The listing builds one solid part. Answer for the finished solid, in the listing's coordinates (mm). A direction names the side the tool comes from. Give positions to 0.01 mm unless a question says otherwise; leave off trailing zeros. Loops run counter-clockwise (first coordinate to the right, second up) from the corner with the lowest first, then second, coordinate; pieces in that order, holes last. Notation, with made-up numbers: M 64,0.25 L 110,0.25 A19 cw 110,18.25 Z; hole C 88,28 d10. An arc over 180 degrees is marked long. One line per item, written item: value. Start each with the question number.
Q1. Flat-ended cylindrical pins translate along their axes: pin 1 (0.5 mm diameter, centred on x = -13, y = 32, fed in from +Z); pin 2 (0.8 mm diameter, centred on x = 112.5, y = 6.5, fed in from -Z). Find the tip coordinate at first contact, or state that the pin passes through.
Q2. For faces 4 (the flat face through (42, 31.143, 4)), 5 (the flat face through (41, 32.768, 0)), determine the directions among +Z, -Z, +X, -X, +Y, -Y from which every point of the face is accessible in a straight line to the end or side of a thin tool.
Q3. The mould has two halves that part along X. Classify faces 1 (the flat face through (117.416, 6, 0)), 2 (the flat face through (41, 7, -25)), 3 (the flat face through (42, -18.794, 4)): +X half, -X half, draft (parallel to the pull), parting line (faces both ways), or undercut.
Q4. A cutting plane is placed at C-C, the plane y = 24. Determine the outline of the cut face in (x, z), and give its area (3 significant figures).
Q5. Consider L1, parallel to Y at x = 104.5, z = 12; L2, parallel to Z at x = 64.5, y = 27.5; L3, parallel to X at y = -1.5, z = 22.5. Determine where each line is inside the solid, lowest interval first.
Q6. A cutting plane is placed at D-D, the plane x = -11.5. Determine the outline of the cut face in (y, z).
Q7. A cutting plane is placed at B-B, the plane z = 17. State how many separate pieces and enclosed holes the cut face has, and give its area (3 significant figures).
Q8. A cutting plane is placed at A-A, the plane x = 88. Determine the outline of the cut face in (y, z), and give its area (3 significant figures).
from build123d import *

# Parameters (mm, degrees)
SKETCH_1_W                = 150
SKETCH_1_H                = 53.201915286
EXTRUDE_1_DEPTH           = 25
CUT_EXTRUDE_4_DEPTH       = 132.308761728
CUT_EXTRUDE_4_DEPTH_BACK  = 132.308761728
SKETCH_2_W                = 13.960564471
SKETCH_2_H                = 10.187423892
SKETCH_2_W_2              = 14
SKETCH_2_W_3              = 12
SKETCH_2_H_2              = 5
SKETCH_4_W                = 147.277496434
SKETCH_4_H                = 49.937069792
CUT_EXTRUDE_9_DEPTH       = 40
EXTRUDE_2_DEPTH           = 0.1
EXTRUDE_2_DEPTH_BACK      = 2
SKETCH_6_W                = 147.277496434
SKETCH_6_H                = 49.937069792
CUT_EXTRUDE_11_DEPTH      = 132.012543018
CUT_EXTRUDE_11_DEPTH_BACK = 0.1
SKETCH_7_R                = 0.5


with BuildPart() as part:
    # 草图1 → 凸台-拉伸1 (new, symmetric)
    with BuildSketch(Plane.XY):
        with Locations((42.416128008, 6.167004021)):
            Rectangle(SKETCH_1_W, SKETCH_1_H)
    extrude(amount=EXTRUDE_1_DEPTH, both=True)

    # 草图2 → 切除-拉伸4 (cut, two sides: drawn at the far end of the back side and taken through both)
    with BuildSketch(Plane(origin=(0, 32.767961664, 0), x_dir=(1, 0, 0), z_dir=(0, 1, 0)).offset(-CUT_EXTRUDE_4_DEPTH_BACK)):
        with Locations((-15.114618297, -19.093711946)):
            Rectangle(SKETCH_2_W, SKETCH_2_H)
        with Locations((5.995879761, -19.093711946)):
            Rectangle(SKETCH_2_W_2, SKETCH_2_H)
        with Locations((99.312670009, -16.792388629)):
            Rectangle(SKETCH_2_W_3, SKETCH_2_H_2)
    extrude(amount=CUT_EXTRUDE_4_DEPTH + CUT_EXTRUDE_4_DEPTH_BACK, mode=Mode.SUBTRACT)

    # 草图4 → 切除-拉伸9 (cut)
    with BuildSketch(Plane.XY.offset(25)):
        with Locations((42.684765752, 6.174377474)):
            Rectangle(SKETCH_4_W, SKETCH_4_H)
    extrude(amount=-CUT_EXTRUDE_9_DEPTH, mode=Mode.SUBTRACT)

    # 草图6 → 凸台-拉伸2 (add, two sides: drawn at the far end of the back side and taken through both)
    with BuildSketch(Plane.XY.offset(25).offset(-EXTRUDE_2_DEPTH_BACK)):
        with Locations((42.684765752, 6.174377474)):
            Rectangle(SKETCH_6_W, SKETCH_6_H)
    extrude(amount=EXTRUDE_2_DEPTH + EXTRUDE_2_DEPTH_BACK)

    # 草图7 → 切除-拉伸11 (cut, two sides: drawn at the far end of the back side and taken through both)
    with BuildSketch(Plane(origin=(0, 0, 23), x_dir=(-1, 0, 0), z_dir=(0, 0, -1)).offset(-CUT_EXTRUDE_11_DEPTH_BACK)):
        with Locations((-112.698705999, 6.167004021)):
            Circle(SKETCH_7_R)
        with Locations((27.866449983, 6.174377474)):
            Circle(SKETCH_7_R)
    extrude(amount=CUT_EXTRUDE_11_DEPTH + CUT_EXTRUDE_11_DEPTH_BACK, mode=Mode.SUBTRACT)


solid = part.part
Answer block:
1. pin 1: z = 25
1. pin 2: z = -25
2. face 4: none
2. face 5: +Z, -Z, +X, -X, +Y
3. face 1: +X half
3. face 2: draft
3. face 3: undercut
4. outline: M -32.58,-25 L 117.42,-25 L 117.42,25 L 116.32,25 L 116.32,25.1 L -30.95,25.1 L -30.95,25 L -32.58,25 Z; hole M -30.95,-15 L 116.32,-15 L 116.32,23 L -30.95,23 Z
4. area: 1,920 mm^2
5. L1: -20.43 to -18.79, 31.14 to 32.77
5. L2: -25 to -15, 23 to 25.1
5. L3: -32.58 to -30.95, 116.32 to 117.42
6. outline: M -20.43,-25 L 32.77,-25 L 32.77,14 L 31.14,14 L 31.14,-15 L -18.79,-15 L -18.79,14 L -20.43,14 Z; M -20.43,24.19 L -18.79,24.19 L -18.79,23 L 31.14,23 L 31.14,24.19 L 32.77,24.19 L 32.77,25 L 31.14,25 L 31.14,25.1 L -18.79,25.1 L -18.79,25 L -20.43,25 Z
7. separate pieces: 6
7. enclosed holes: 0
7. area: 495 mm^2
8. outline: M -20.43,-25 L 32.77,-25 L 32.77,25 L 31.14,25 L 31.14,25.1 L -18.79,25.1 L -18.79,25 L -20.43,25 Z; hole M -18.79,-15 L 31.14,-15 L 31.14,23 L -18.79,23 Z
8. area: 767 mm^2
